Verification items for this drawing (mm, ordinates from the low corner). A direction names the side the tool comes from. Coordinates: 2 decimals unless noted, no trailing zeros. Order: outer loops, then holes, each group sorted by start corner. A loop starts at its lowest first (then second) coordinate and runs counter-clockwise, first axis right, second up. Notation, with made-up numbers: (33.25, 50.25) -> (67.25, 50.25) arc R32 ccw to (67.25, 88.25) -> close; hole circle Ø3 at (13.5, 58). An arc over 180 degrees is marked (long way). Answer as CSV lines item,"result". Start each with the question number.
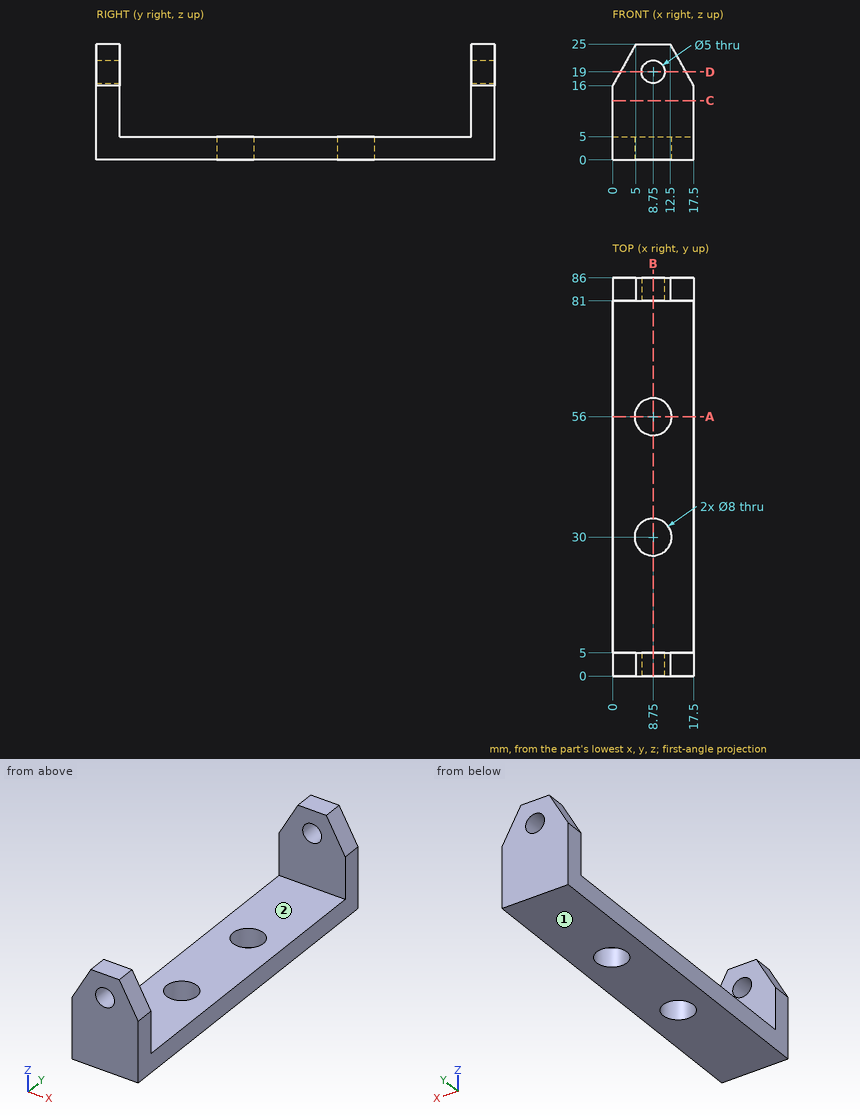
Q1. Access from +Z, -Z, +X, -X, +Y, -Y to the whole of each face (thin tool, end or side, straight path). Record for the marked faces 1 and 2.
Q2. Thickness scan on L1, parallel to Y at x = 8.75, z = 2.65; L2, parallel to Z at x = 8.75, y = 1.35; L3, parallel to Y at x = 11.25, z = 19.5. Record the ranges inside material, lowest first.
Q3. Sectioned sample at A-A, the plane y = 56. Record the cut outline in (x, z).
Q4. Sectioned sample at D-D, the plane z = 19. Record the cut outline in (x, y), then the cut area to 3 significant figures.
Q5. Sectioned sample at B-B, the plane x = 8.75. Record the cut outline in (y, z).
Q6. Go/stop test with flat-tipped pins: pin 1 Ø9 at (x, y) = (8.75, 56) entering from +Z; pin 2 Ø7 at (x, y) = (8.75, 30) entering from +Z. Record where each tip stops, or that it passes through.
Q7. Sectioned sample at C-C, the plane z = 12.75. Record the cut outline in (x, y), then the cut area to 3 significant figures.
Geometry results:
1,face 1,"-Z, +X, -X, +Y, -Y"
1,face 2,"+Z, +X, -X"
2,L1,"y = 0 to 26, 34 to 52, 60 to 86"
2,L2,"z = 0 to 16.5, 21.5 to 25"
2,L3,"y = 0 to 5, 81 to 86"
3,outline,"(0, 0) -> (4.75, 0) -> (4.75, 5) -> (0, 5) -> close; (12.75, 0) -> (17.5, 0) -> (17.5, 5) -> (12.75, 5) -> close"
4,outline,"(1.67, 0) -> (6.25, 0) -> (6.25, 5) -> (1.67, 5) -> close; (1.67, 81) -> (6.25, 81) -> (6.25, 86) -> (1.67, 86) -> close; (11.25, 0) -> (15.83, 0) -> (15.83, 5) -> (11.25, 5) -> close; (11.25, 81) -> (15.83, 81) -> (15.83, 86) -> (11.25, 86) -> close"
4,area,"91.7 mm^2"
5,outline,"(0, 0) -> (26, 0) -> (26, 5) -> (5, 5) -> (5, 16.5) -> (0, 16.5) -> close; (0, 21.5) -> (5, 21.5) -> (5, 25) -> (0, 25) -> close; (34, 0) -> (52, 0) -> (52, 5) -> (34, 5) -> close; (60, 0) -> (86, 0) -> (86, 16.5) -> (81, 16.5) -> (81, 5) -> (60, 5) -> close; (81, 21.5) -> (86, 21.5) -> (86, 25) -> (81, 25) -> close"
6,pin 1,"stops at z = 5"
6,pin 2,"passes through"
7,outline,"(0, 0) -> (17.5, 0) -> (17.5, 5) -> (0, 5) -> close; (0, 81) -> (17.5, 81) -> (17.5, 86) -> (0, 86) -> close"
7,area,"175 mm^2"
